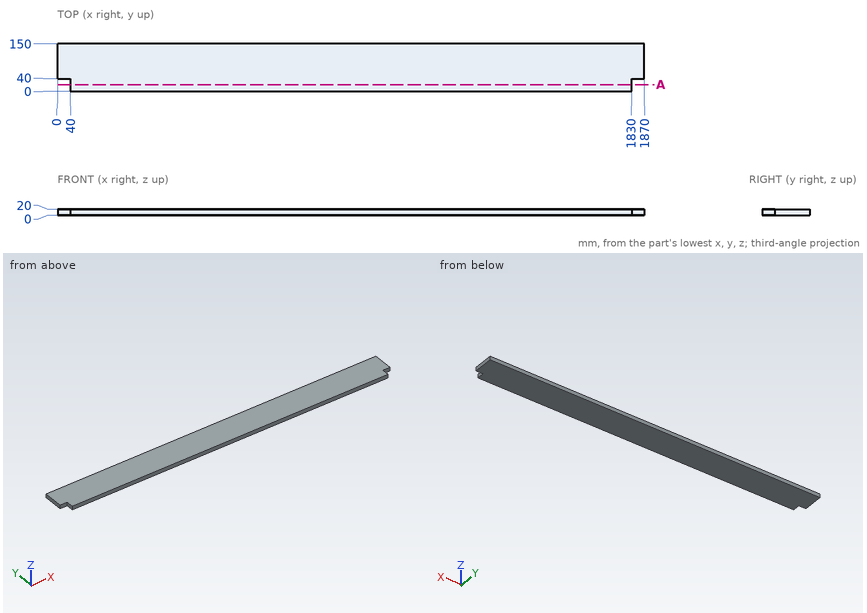
Can you work these out from the drawing? Everything is in mm from the part's minimum corner. Round coordinates to 2 decimals unless told otherwise and drop trailing zeros. Order: outer loops, then holes, each group sorted by start corner. A loop starts at its lowest first (then second) coordinate and runs counter-clockwise, first axis right, second up. Notation, with made-up numbers: M 50.25,13.25 L 90.25,13.25 A23 cw 90.25,43.25 Z; hole C 5,-24.5 d5. An arc over 180 degrees is marked long. Answer as CSV lines item,"result".
Item 1: For pin 1 (6 mm diameter, centred on y = 28, z = 8, fed in from +X); pin 2 (6 mm diameter, centred on y = 28.5, z = 6.5, fed in from -X); pin 3 (6 mm diameter, centred on x = 1851, z = 8.5, fed in from -Y), each with a flat end and sliding along its axis, tell me the tip position at first contact or that it passes through.
From the geometry:
pin 1,"x = 1830"
pin 2,"x = 40"
pin 3,"y = 40"
Item 2: Please list where this line runs through material, in increasing order: L1, parallel to X at y = 9, z = 14.5. Write a range as [from, to].
From the geometry:
L1,"[40, 1830]"
Item 3: Imagine slicing it at A-A on y = 20.5. List the corners of the cut face in (x, z) for me.
From the geometry:
outline,"M 40,0 L 1830,0 L 1830,20 L 40,20 Z"
